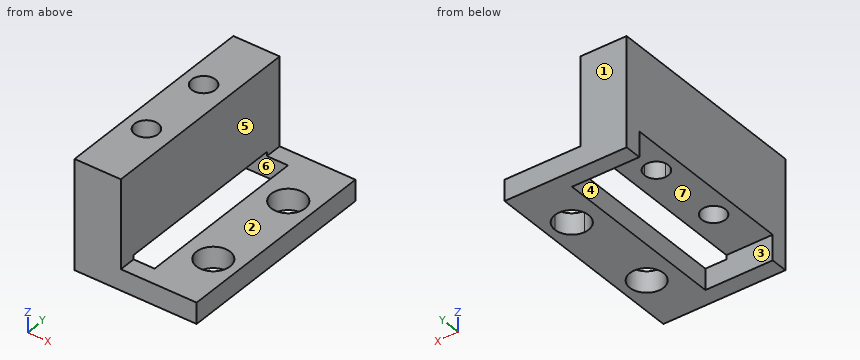
```python
from build123d import *

# Parameters (mm, degrees)
F0_R     = 2
F1_DEPTH = 2.5
F2_R     = 1.405868
F3_DEPTH = 13
F4_W     = 8.5
F4_H     = 21
F5_DEPTH = 3


with BuildPart() as f1:
    # F0 (on Top) → F1 (new body)
    with BuildSketch(Plane.XY):
        with BuildLine():
            ThreePointArc((35.5, 18.4), (32.085786, 19.814214), (33.5, 16.4))
            ThreePointArc((33.5, 16.4), (34.914214, 16.985786), (35.5, 18.4))
        make_face()
        Polygon((26, 12.5), (26, 0), (36.5, 0), (36.5, 25), (26, 25), align=None)
        with Locations((33.5, 6.6)):
            Circle(F0_R, mode=Mode.SUBTRACT)
        with BuildLine():
            ThreePointArc((35.5, 18.4), (34.914214, 16.985786), (33.5, 16.4))
            ThreePointArc((33.5, 16.4), (32.085786, 19.814214), (35.5, 18.4))
        make_face(mode=Mode.SUBTRACT)
    extrude(amount=F1_DEPTH)

    # F2 (on Top) → F3 (join)
    with BuildSketch(Plane.XY):
        with BuildLine():
            ThreePointArc((25.905868, 17), (23.505901, 17.994099), (24.5, 15.594132))
            ThreePointArc((24.5, 15.594132), (25.494099, 16.005901), (25.905868, 17))
        make_face()
        Polygon((22, 12.5), (22, 0), (27.5, 0), (27.5, 25), (22, 25), align=None)
        with Locations((24.5, 8)):
            Circle(F2_R, mode=Mode.SUBTRACT)
        with BuildLine():
            ThreePointArc((25.905868, 17), (25.494099, 16.005901), (24.5, 15.594132))
            ThreePointArc((24.5, 15.594132), (23.505901, 17.994099), (25.905868, 17))
        make_face(mode=Mode.SUBTRACT)
    extrude(amount=F3_DEPTH)

    # F4 (on Top) → F5 (cut)
    with BuildSketch(Plane.XY):
        with Locations((25.75, 12.5)):
            Rectangle(F4_W, F4_H)
    extrude(amount=F5_DEPTH, mode=Mode.SUBTRACT)


solid = f1.part
```
Here's how the part is built. I have some questions about the finished solid (model axes, mm). Face numbers are marked on the shaded views. A direction names the side the tool comes from. Coordinates: 2 decimals unless noted, no trailing zeros. Order: outer loops, then holes, each group sorted by start corner. A loop starts at its lowest first (then second) coordinate and runs counter-clockwise, first axis right, second up. Notation, with made-up numbers: M -34.75,17 L 9.25,17 A24 cw 9.25,42 Z; hole C 22.25,55.5 d2. An arc over 180 degrees is marked long. Answer as a JSON object with one key per item and string values. Group by question number.
(1) For pin 1 (1 mm diameter, centred on y = 17, z = 3.5, fed in from +X); pin 2 (3 mm diameter, centred on x = 24.5, y = 17, fed in from -Z); pin 3 (7 mm diameter, centred on x = 32.5, y = 12.5, fed in from +Z), each with a flat end and sliding along its axis, tell me the tip position at first contact or that it passes through.
(2) Suppose I cut it at D-D, the plane y = 8. Please give me the cut outline in (x, z), then the cut area to 3 significant figures.
(3) Suppose I cut it at C-C, the plane y = 19.5. Please give me the cut outline in (x, z).
(4) Suppose I cut it at A-A, the plane z = 7. Please give me the cut outline in (x, y).
(5) I need wall thicknesses on probe 1 along Y at (x, z) = (24.5, 10.75); probe 2 along Y at (x, z) = (33.5, 1.65); probe 3 along X at (y, z) = (17, 6.5). Which ranges of each line are inside material? Lowest first, please.
(6) If we mould it in two halves opening along Y, with no side actions, what happens to the marked faces 1, 2 and 3? For each: released by +Y, released by -Y, zero draft, split by the parting line, or undercut.
(7) Which directions (+Z, -Z, +X, -X, +Y, -Y) give clear straight access to the entire face, cutting with the end or side of a thin tool? Please do the marked faces 4, 5, 6 and 7.
(8) Suppose I cut it at B-B, the plane x = 28.5. Please give me the cut outline in (y, z).
Values found:
{
 "1": {"pin 1": "stops at x = 27.5", "pin 2": "stops at z = 3", "pin 3": "stops at z = 2.5"},
 "2": {"outline": "M 22,3 L 23.09,3 L 23.09,13 L 22,13 Z; M 25.91,3 L 27.5,3 L 27.5,13 L 25.91,13 Z; M 30,0 L 32.07,0 L 32.07,2.5 L 30,2.5 Z; M 34.93,0 L 36.5,0 L 36.5,2.5 L 34.93,2.5 Z", "area": "36.0 mm^2"},
 "3": {"outline": "M 22,3 L 27.5,3 L 27.5,13 L 22,13 Z; M 30,0 L 31.83,0 L 31.83,2.5 L 30,2.5 Z; M 35.17,0 L 36.5,0 L 36.5,2.5 L 35.17,2.5 Z"},
 "4": {"outline": "M 22,0 L 27.5,0 L 27.5,25 L 22,25 Z; hole C 24.5,8 d2.81; hole C 24.5,17 d2.81"},
 "5": {"probe 1": "y = 0 to 6.59, 9.41 to 15.59, 18.41 to 25", "probe 2": "y = 0 to 4.6, 8.6 to 16.4, 20.4 to 25", "probe 3": "x = 22 to 23.09, 25.91 to 27.5"},
 "6": {"face 1": "released by +Y", "face 2": "zero draft", "face 3": "undercut"},
 "7": {"face 4": "+Z, -Z, -X", "face 5": "+Z, +X, +Y, -Y", "face 6": "-Z, -X", "face 7": "-Z, +X, -X"},
 "8": {"outline": "M 0,0 L 2,0 L 2,2.5 L 0,2.5 Z; M 23,0 L 25,0 L 25,2.5 L 23,2.5 Z"}
}
